Autodesk Inventor part; units mm, degrees
ref_plane "YZ Plane" through (0, 0, 0) normal (1, 0, 0) x (0, 1, 0)
ref_plane "XZ Plane" through (0, 0, 0) normal (0, 1, 0) x (-1, 0, 0)
ref_plane "XY Plane" through (0, 0, 0) normal (0, 0, 1) x (1, 0, 0)
sketch "Sketch1" plane through (0, 0, 0) normal (0, 1, 0) x (-1, 0, 0)
  line L0 (0, 0) -> (0, 98.679)
  line L1 (0, 0) -> (98.679, 0) construction
  line L2 (0, 98.679) -> (0, -98.679)
  line L3 (0, 98.679) -> (4, 98.679)
  line L4 (4, 98.679) -> (4, -98.679)
  line L5 (4, -98.679) -> (0, -98.679)
  line L6 (4, -98.679) -> (4, -102.679)
  line L7 (4, -102.679) -> (0, -102.679)
  line L8 (0, -102.679) -> (0, -98.679)
  line L9 (4, 98.679) -> (4, 102.679)
  line L10 (4, 102.679) -> (0, 102.679)
  line L11 (0, 102.679) -> (0, 98.679)
  dimension "d0" = 98.679
  dimension "d1" = 90
  dimension "d2" = 197.358
  dimension "d3" = 4
  dimension "d4" = 4
  dimension "d5" = 4
extrude "Extrusion3" add sketch "Sketch1" along normal blind 4 contours L0 L3 L4 L5 L2
extrude "Extrusion4" add sketch "Sketch1" along normal blind 30 contours L11 L10 L9 L3 | L5 L6 L7 L8
sketch "Sketch3" plane through (0, 4, 0) normal (0, 1, 0) x (1, 0, 0)
  line L0 (-4, 102.679) -> (-4, -102.679)
  line L1 (-4, -102.679) -> (-2, -102.679)
  line L2 (-2, -102.679) -> (-2, 0)
  point P0 (0, 0)
  dimension "d15" = 2
hole "Hole1" at (-2, 4, 0) direction (0, -1, 0) diameter 3.4 end through all
Check sheet for the modelled part. Datum: model origin and axes. Units: mm. A direction names the side the tool comes from. Give positions to 0.01 mm unless a question says otherwise; leave off trailing zeros. Order: outer loops, then holes, each group sorted by start corner. A loop starts at its lowest first (then second) coordinate and runs counter-clockwise, first axis right, second up. Notation, with made-up numbers: (-34, 13) -> (13, 13) arc R30 ccw to (13, 38) -> close; hole circle Ø5 at (72.25, -23.5). An arc over 180 degrees is marked (long way). Use CSV: the item, a comma, the result in double quotes. Start each with the question number.
1) Sectioned sample at A-A, the plane y = 27.75. Record the boundary of the cut face in (x, z).
2) Sectioned sample at D-D, the plane z = 32. Record the boundary of the cut face in (x, y).
3) Mould release check, pull along X, two halves, no side actions. Record for faces 3 (the face through (-3.15, 1.97, -1.25)), 4 (the face through (-2, 30, -101)), 5 (the face through (0, 3.8, -15.7)), 6 (the face through (-4, 3.8, 15.7)): released by +X, released by -X, zero draft, split by the parting line, or undercut.
4) Material ranges on line 1 (Z direction, x = -0.5, y = 7.5); line 2 (Z direction, x = -2, y = 1.75); line 3 (X direction, y = 2.4, z = 0), recorded low to high. Write a range as from..to.
5) Go/stop test with a flat-tipped pin: P1, Ø1.2, axis at x = -1.5, z = -6, coming from the +Y side. Record where the tip stops, or that it passes through.
6) Sectioned sample at C-C, the plane z = 0. Record the boundary of the cut face in (x, y), plus the area to 3 significant figures.
7) Sectioned sample at B-B, the plane x = -2. Record the boundary of the cut face in (y, z), plus the area to 3 significant figures.
8) Set-up check for faces 1 (the face through (-3.3, 4, 1.4)), 2 (the face through (-2, 15, -102.679)): record each of +Z, -Z, +X, -X, +Y, -Y from which the full face is reachable in a straight line by a thin tool's end or side.
Recorded:
1,outline,"(-4, -102.68) -> (0, -102.68) -> (0, -98.68) -> (-4, -98.68) -> close; (-4, 98.68) -> (0, 98.68) -> (0, 102.68) -> (-4, 102.68) -> close"
2,outline,"(-4, 0) -> (0, 0) -> (0, 4) -> (-4, 4) -> close"
3,face 3,"undercut"
3,face 4,"zero draft"
3,face 5,"released by +X"
3,face 6,"released by -X"
4,line 1,"-102.68..-98.68, 98.68..102.68"
4,line 2,"-102.68..-1.7, 1.7..102.68"
4,line 3,"-4..-3.7, -0.3..0"
5,P1,"y = 4"
6,outline,"(-4, 0) -> (-3.7, 0) -> (-3.7, 4) -> (-4, 4) -> close; (-0.3, 0) -> (0, 0) -> (0, 4) -> (-0.3, 4) -> close"
6,area,"2.40 mm2"
7,outline,"(0, -102.68) -> (30, -102.68) -> (30, -98.68) -> (4, -98.68) -> (4, -1.7) -> (0, -1.7) -> close; (0, 1.7) -> (4, 1.7) -> (4, 98.68) -> (30, 98.68) -> (30, 102.68) -> (0, 102.68) -> close"
7,area,"1,020 mm2"
8,face 1,"+X, -X, +Y"
8,face 2,"-Z, +X, -X, +Y, -Y"
